Check sheet for the drawn part. Datum: minimum x, y, z corner. Units: mm. A direction names the side the tool comes from. Round coordinates to 2 decimals unless told otherwise and drop trailing zeros. Write each loop counter-clockwise with the first axis right and the second up, starting at its lowest first coordinate (ties: lowest second). Pieces come first, ordered by that corner, then holes.
Item 1: Cross-section at A-A on y = 9.5. Enter the section's corners in (x, z) (1 decimal).
Item 2: Cross-section at D-D on z = 9.5. Enter the section's corners in (x, y) (3 decimals), plus the area to 3 significant figures.
Item 3: Tool access check on the marked faces 1 and 2. Record the directions out of +Z, -Z, +X, -X, +Y, -Y that give a thin tool (end or side, any length) a straight path to the whole face; none if there is none.
Item 4: Cross-section at C-C on x = 2.55. Count the separate pieces of the cut face and the enclosed holes in it.
Item 5: Release check for a two-part mould opening along Z. For the marked faces 3, 4 and 5 record: +Z half, -Z half, draft (parallel to the pull), parting line (faces both ways), or undercut.
Item 6: Go/stop test with flat-tipped pins: pin 1 Ø1 at (x, z) = (2.5, 5) entering from -Y; pin 2 Ø1.5 at (x, z) = (2, 6) entering from +Y; pin 3 Ø1.5 at (x, z) = (3, 15.5) entering from +Y. Record where each tip stops, or that it passes through.
Item 7: Cross-section at B-B on z = 15.25. Enter the section's corners in (x, y) (1 decimal).
Item 8: Material ranges on line 1 (Z direction, x = 2.2, y = 9.5); line 2 (Z direction, x = 1, y = 10); line 3 (Z direction, x = 2.85, y = 11.5), recorded low to high.
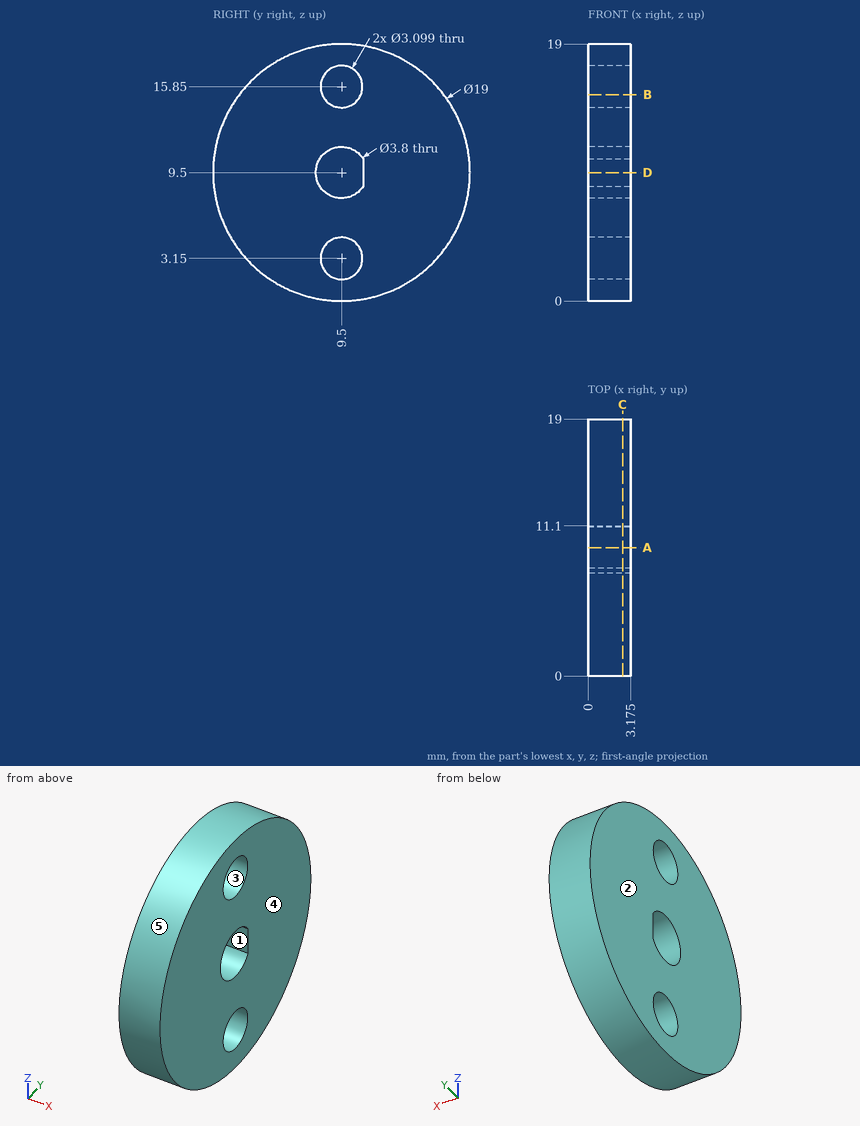
Response values:
1. outline: (0, 0) - (3.2, 0) - (3.2, 1.6) - (0, 1.6) - close; (0, 4.7) - (3.2, 4.7) - (3.2, 7.6) - (0, 7.6) - close; (0, 11.4) - (3.2, 11.4) - (3.2, 14.3) - (0, 14.3) - close; (0, 17.4) - (3.2, 17.4) - (3.2, 19) - (0, 19) - close
2. outline: (0, 0) - (3.175, 0) - (3.175, 7.6) - (0, 7.6) - close; (0, 11.1) - (3.175, 11.1) - (3.175, 19) - (0, 19) - close
2. area: 49.2 mm2
3. face 1: +X, -X
3. face 2: +Z, -Z, -X, +Y, -Y
4. separate pieces: 1
4. enclosed holes: 3
5. face 3: undercut
5. face 4: draft
5. face 5: parting line
6. pin 1: stops at y = 0.88
6. pin 2: stops at y = 18.59
6. pin 3: stops at y = 17.42
7. outline: (0, 1.9) - (3.2, 1.9) - (3.2, 8.1) - (0, 8.1) - close; (0, 10.9) - (3.2, 10.9) - (3.2, 17.1) - (0, 17.1) - close
8. line 1: z = 0 to 1.6, 4.7 to 7.6, 11.4 to 14.3, 17.4 to 19
8. line 2: z = 0.01 to 1.68, 4.62 to 7.67, 11.33 to 14.38, 17.32 to 18.99
8. line 3: z = 0.21 to 18.79
